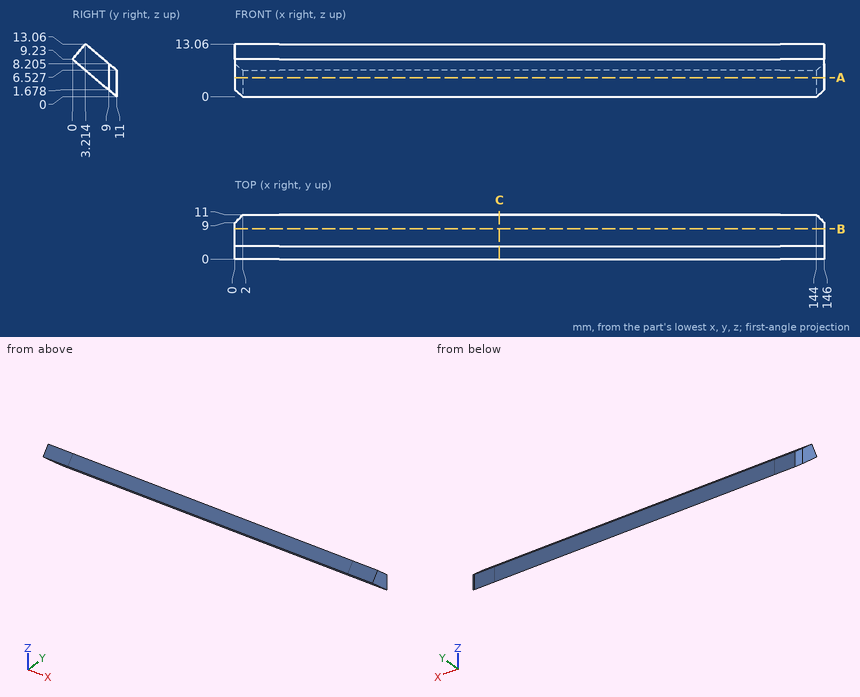
Design review of the part shown in the three views and the two pictorial views. Dimensions are in mm from the part's minimum x, y and z. Round coordinates to 2 decimals unless told otherwise and drop trailing zeros. Order: outer loops, then holes, each group sorted by start corner. A loop starts at its lowest first (then second) coordinate and runs counter-clockwise, first axis right, second up.
Item 1: Add section C-C, the plane x = 65.5. State the section outline as (y, z) points, and give its area (3 significant figures).
Working result:
outline: (0, 9.23) - (11, 0) - (11, 6.53) - (3.21, 13.06) - close
area: 61.3 mm2
Item 2: Add section A-A, the plane z = 4.75. State the section outline as (x, y) points.
Working result:
outline: (0, 5.34) - (146, 5.34) - (146, 9) - (144, 11) - (11, 11) - (2, 11) - (0, 9) - close
Item 3: To check wall thickness, follow probe 1 along Y at (x, z) = (80.5, 3.75); probe 2 along Z at (x, y) = (114, 9) (1 decimal); probe 3 along Y at (x, z) = (71, 12) (1 decimal). State the ranges of each line that lie inside material, in increasing order.
Working result:
probe 1: y = 6.53 to 11
probe 2: z = 1.7 to 8.2
probe 3: y = 2.3 to 4.5
Item 4: For pin 1 (4 mm diameter, centred on x = 57, y = 8, fed in from -Z); pin 2 (1 mm diameter, centred on x = 81, y = 5, fed in from -Z) (1 decimal); pin 3 (2 mm diameter, centred on x = 34, z = 8.5, fed in from +Y), all flat-tipped, find the tip position at first contact; note any pin that passes through.
Working result:
pin 1: stops at z = 0.84
pin 2: stops at z = 4.6
pin 3: stops at y = 9.84
Item 5: Add section B-B, the plane y = 7.5. State the section outline as (x, z) points.
Working result:
outline: (0, 2.94) - (146, 2.94) - (146, 9.46) - (0, 9.46) - close
